```python
from build123d import *

# Parameters (mm, degrees)
SKETCH1_R             = 95
BOSS_EXTRUDE1_DEPTH   = 19
SKETCH2_R             = 27.5
CUT_EXTRUDE1_DEPTH    = 136.687140142
SKETCH3_R             = 1.730453225
CUT_EXTRUDE2_DEPTH    = 14.244742
CIRPATTERN1_START     = 4.755257679
CIRPATTERN1_OUTLINE_R = 1.730453225
CIRPATTERN1_DEPTH     = 14.244742321


# Read off the part's stored shape, not the designer's step: CirPattern1
with BuildPart() as part:
    # Sketch1 → Boss-Extrude1 (new body)
    with BuildSketch(Plane(origin=(0, 0, 0), x_dir=(1, 0, 0), z_dir=(0, 1, 0))):
        with Locations(Location((0, 0, 0), (0, 0, 270))):
            Circle(SKETCH1_R)
    extrude(amount=BOSS_EXTRUDE1_DEPTH)

    # Sketch2 → Cut-Extrude1 (cut, through all)
    with BuildSketch(Plane(origin=(0, 0, 0), x_dir=(1, 0, 0), z_dir=(0, 1, 0))):
        with Locations(Location((0, 0, 0), (0, 0, 270))):
            Circle(SKETCH2_R)
    extrude(amount=CUT_EXTRUDE1_DEPTH, mode=Mode.SUBTRACT)

    # Sketch3 → Cut-Extrude2 (cut)
    with BuildSketch(Plane(origin=(0, 19, 0), x_dir=(1, 0, 0), z_dir=(0, 1, 0))):
        with Locations(Location((-32.655618967, 0, 0), (0, 0, 270))):
            Circle(SKETCH3_R)
    extrude(amount=-CUT_EXTRUDE2_DEPTH, mode=Mode.SUBTRACT)

    # CirPattern1 outline → CirPattern1 (cut)
    with BuildSketch(Plane(origin=(0, 0, 0), x_dir=(1, 0, 0), z_dir=(0, 1, 0)).offset(CIRPATTERN1_START)):
        with Locations((-10.091141223, 31.057339213)):
            Circle(CIRPATTERN1_OUTLINE_R)
        with Locations((26.418950707, 19.194491234)):
            Circle(CIRPATTERN1_OUTLINE_R)
        with Locations((26.418950707, -19.194491234)):
            Circle(CIRPATTERN1_OUTLINE_R)
        with Locations((-10.091141223, -31.057339213)):
            Circle(CIRPATTERN1_OUTLINE_R)
    extrude(amount=CIRPATTERN1_DEPTH, mode=Mode.SUBTRACT)


solid = part.part
```
Design review of the part built by this model. Coordinates are the model's own, in mm. Give positions to 0.01 mm unless a question says otherwise; leave off trailing zeros. Loops run counter-clockwise (first coordinate to the right, second up) from the corner with the lowest first, then second, coordinate; pieces in that order, holes last. Notation, with made-up numbers: M 79.25,45 L 106.25,45 A4 ccw 106.25,52 Z; hole C -14.5,1 d10. An arc over 180 degrees is marked long. Return JSON: item names as keys, results as strings. Group by question number.
Item 1: We need section D-D (z = -48). Give the boundary of the cut face in (x, y).
Item 2: For probe 1 along X at (y, z) = (8, 0); probe 2 along Z at (x, y) = (-1.5, 12.5); probe 3 along Z at (x, y) = (-14, 9.5), list the stretches that pass through material, from the lowest coordinate up.
Item 3: Insertion check: pin 1 Ø3 at (x, z) = (-10.09, 31.06) entering from +Y; pin 2 Ø6 at (y, z) = (12, -50.5) entering from +X; pin 3 Ø3 at (x, y) = (-19, 6) entering from -Z. Each pin has a flat end and moves straight along its axis. Give the tip position at first contact, or say it passes through.
Item 4: We need section C-C (x = -57). Give the boundary of the cut face in (y, z).
Item 5: We need section A-A (x = 0). Give the boundary of the cut face in (y, z), and give its area (4 significant figures).
Item 6: We need section B-B (y = 12.5). Give the boundary of the cut face in (x, z).
Item 7: Mouldability with a two-part tool opening along X and no side actions: class faces 1 (the flat face through (-20, 19, 20)), 2 (the cylindrical face through (-24.397, 9.367, 12.69)), 3 (the cylindrical face through (-92.74, 9.37, -20.59)) as released by +X, released by -X, zero draft, split by the parting line, or undercut.
Output:
{
 "1": {"outline": "M -81.98,0 L 81.98,0 L 81.98,19 L -81.98,19 Z"},
 "2": {"probe 1": "x = -95 to -34.39, -30.93 to -27.5, 27.5 to 95", "probe 2": "z = -94.99 to -27.46, 27.46 to 94.99", "probe 3": "z = -93.96 to -23.67, 23.67 to 93.96"},
 "3": {"pin 1": "stops at y = 4.76", "pin 2": "stops at x = 82.27", "pin 3": "stops at z = -93.37"},
 "4": {"outline": "M 0,-76 L 19,-76 L 19,76 L 0,76 Z"},
 "5": {"outline": "M 0,-95 L 19,-95 L 19,-27.5 L 0,-27.5 Z; M 0,27.5 L 19,27.5 L 19,95 L 0,95 Z", "area": "2,565 mm^2"},
 "6": {"outline": "C 0,0 d190; hole C -32.66,0 d3.46; hole C 0,0 d55; hole C -10.09,-31.06 d3.46; hole C -10.09,31.06 d3.46; hole C 26.42,-19.19 d3.46; hole C 26.42,19.19 d3.46"},
 "7": {"face 1": "zero draft", "face 2": "undercut", "face 3": "split by the parting line"}
}
